Autodesk Inventor part; units mm, degrees
ref_plane "Work Plane1" through (0, 0, 0) normal (1, 0, 0) x (0, 1, 0)
ref_plane "XZ Plane" through (0, 0, 0) normal (0, 1, 0) x (-1, 0, 0)
ref_plane "XY Plane" through (0, 0, 0) normal (0, 0, 1) x (1, 0, 0)
sketch "Sketch1" plane through (0, 0, 0) normal (0, 0, 1) x (1, 0, 0)
  circle A0 centre (0, 0) radius 0.75
  circle A1 centre (0, 0) radius 4
  dimension "d0" = 1.5
  dimension "d1" = 8
extrude "Extrusion1" add sketch "Sketch1" along normal blind 6 contours A0 | A1
extrude "Extrusion2" cut sketch "Sketch1" along normal blind 4 contours A0
ref_plane "Work Plane1" through (0, 0, 0) normal (1, 0, 0) x (0, 1, 0)
sketch "Sketch2" plane through (0, 0, 0) normal (1, 0, 0) x (0, 1, 0)
  line L0 (1.9777, 1) -> (-1.4864, 3)
  line L1 (1.9777, 1) -> (5.9777, 1) construction
  line L2 (1.9777, 1) -> (1.9777, 3)
  line L3 (1.9777, 3) -> (0.9602, 3.5874)
  line L4 (-4, 0) -> (4, 0)
  line L5 (0.9602, 3.5874) -> (-1.4864, 5)
  line L6 (-1.4864, 5) -> (-1.4864, 3)
  line L7 (-4, 6) -> (4, 6)
  point P0 (0, 0)
  dimension "d7" = 150
  dimension "d8" = 2
  dimension "d9" = 1
  dimension "d10" = 1
extrude "Extrusion3" add sketch "Sketch2" along normal blind 25
sketch "Sketch3" plane through (0, 0, 0) normal (1, 0, 0) x (0, 1, 0)
  point P0 (0, 0)
pattern_circular "Circular Pattern1" count 6 over 360 about axis through (0, 0, 0) along (0, 0, 1) of "Extrusion3"
properties part number "propeler"
Build history of the part. All positions in model axes, mm. A direction names the side the tool comes from. Round coordinates to 2 decimals unless told otherwise and drop trailing zeros. Write each loop counter-clockwise with the first axis right and the second up, starting at its lowest first coordinate (ties: lowest second). Pieces come first, ordered by that corner, then holes. Notation, with made-up numbers: M 20.5,38 L 62.5,38 A15 ccw 62.5,67 Z; hole C -2,37 d3. An arc over 180 degrees is marked long. Answer as a JSON object with one key per item and string values. Group by question number.
(1) Cut at B-B (x = 20). Give the cut face in (y, z), and give its area (3 significant figures).
(2) Mould opens along X. For faces 1 (the flat face through (-5.82, 13.05, 4.01)), 2 (the flat face through (14, 1.978, 2)), 3 (the flat face through (25, 0, 3)) say: pulls with the +X half, pulls with the -X half, needs draft (parallel to the pull), parting line crosses it, or undercut.
(3) Cut at A-A (y = -12). Give the cut face in (x, z).
(4) Drill centre lines: L1, parallel to X at y = 0, z = 0.75; L2, parallel to X at y = -19.5, z = 3.25. Where is each one in solid material? Low to high.
(5) Which spindle directions (+Z, -Z, +X, -X, +Y, -Y) get a long thin tool onto all of the face, cutting with end or side? Do faces 4 (the flat face through (5.33, 13.19, 1.99)), 5 (the flat face through (8.39, 11.56, 4.01)), 6 (the flat face through (6.81, 12.335, 1.986)), 7 (the cylindrical face through (0.69, 0.29, 0.95)). Say none if no direction does.
(6) Flat gauge pins, fed straight in: pin 1 (4 mm diameter, centred on x = -10, y = -14.5, fed in from -Z); pin 2 (5 mm diameter, centred on x = 8, y = 2, fed in from -Z); pin 3 (0.9 mm diameter, centred on x = 0, y = 0, fed in from -Z); pin 4 (8 mm diameter, centred on x = -13.5, y = 8.5, fed in from +Z). Where does each tip first touch, or does it go through?
Responses:
{
 "1": {"outline": "M -1.49,3 L 1.98,1 L 1.98,3 L 0.96,3.59 L -1.49,5 Z", "area": "6.93 mm2"},
 "2": {"face 1": "undercut", "face 2": "needs draft", "face 3": "pulls with the +X half"},
 "3": {"outline": "M -8.64,3 L -4.64,1 L -4.64,3 L -5.82,3.59 L -8.64,5 Z; M 5.21,3 L 9.21,1 L 9.21,3 L 8.04,3.59 L 5.21,5 Z"},
 "4": {"L1": "x = -4 to -0.75, 0.75 to 4", "L2": "x = -12.97 to -9.47, 9.54 to 13.04"},
 "5": {"face 4": "+Z, -Z, +Y", "face 5": "+Z, -Z, +X", "face 6": "-Z, +X", "face 7": "-Z"},
 "6": {"pin 1": "stops at z = 1.8", "pin 2": "stops at z = 1", "pin 3": "stops at z = 1.88", "pin 4": "passes through"}
}
